```python
from build123d import *

# Parameters (mm, degrees)
F0_R     = 3.6
F0_R_2   = 11.05
F1_DEPTH = 6.5


# Not quite as in the source:
# - a feature names something its author has since deleted; it is built from what else it names


with BuildPart() as f1:
    # F0 (on Top) → F1 (new body)
    with BuildSketch(Plane.XY):
        with BuildLine():
            ThreePointArc((-23.0209464524, -29.3076083822), (-19.9383676627, -26.8167802289), (-17.6773098575, -23.5619170235))
            ThreePointArc((-17.6773098575, -23.5619170235), (-20.4709038775, -26.3215082368), (-23.0209464524, -29.3076083822))
        make_face()
        with BuildLine():
            ThreePointArc((-2.5600533635, -14.3957456382), (-1.63787321, -14.0667717582), (-0.7089513801, -13.7573460272))
            ThreePointArc((-0.7089513801, -13.7573460272), (-3.7381834506, -13.2395644299), (-6.5814605839, -12.0733226612))
            Line((-6.5814605839, -12.0733226612), (-2.5600533635, -14.3957456382))
        make_face()
        with BuildLine():
            ThreePointArc((-0.7089513801, -13.7573460272), (3.2568779095, -13.4262355322), (6.9693155956, -11.9926238203))
            ThreePointArc((6.9693155956, -11.9926238203), (3.0926272048, -12.7115843783), (-0.7089513801, -13.7573460272))
        make_face()
        with BuildLine():
            ThreePointArc((29.002813969, -3.3554863963), (22.1605329653, -5.9872334975), (17.5863384821, -11.7160769207))
            ThreePointArc((17.5863384821, -11.7160769207), (17.1389450218, -21.6742013703), (23.4307313902, -29.4058136055))
            ThreePointArc((23.4307313902, -29.4058136055), (37.4314802249, -29.4071108103), (44.4322291397, -17.282322802))
            ThreePointArc((44.4322291397, -17.282322802), (39.8127458528, -6.8897337985), (29.002813969, -3.3554863963))
        make_face()
        with Locations((24.2079713773, -13.6886037443)):
            Circle(F0_R, mode=Mode.SUBTRACT)
        with Locations((36.4874702709, -20.9787380615)):
            Circle(F0_R, mode=Mode.SUBTRACT)
        with Locations((33.9983616409, -11.0225966846)):
            Circle(F0_R, mode=Mode.SUBTRACT)
        with BuildLine():
            ThreePointArc((-23.0209464524, -29.3076083822), (-20.4709038775, -26.3215082368), (-17.6773098575, -23.5619170235))
            ThreePointArc((-17.6773098575, -23.5619170235), (-16.5669328393, -20.5090534106), (-16.1900430763, -17.2824658218))
            ThreePointArc((-16.1900430763, -17.2824658218), (-16.8601676515, -13.0029306649), (-18.8063889562, -9.1330843193))
            ThreePointArc((-18.8063889562, -9.1330843193), (-27.0153338433, -3.6471725985), (-36.8032431016, -4.9428716054))
            ThreePointArc((-36.8032431016, -4.9428716054), (-42.3755818337, -24.1754075155), (-23.0209464524, -29.3076083822))
        make_face()
        with Locations((-26.552398323, -23.5003339555)):
            Circle(F0_R, mode=Mode.SUBTRACT)
        with Locations((-36.419223994, -20.6778945734)):
            Circle(F0_R, mode=Mode.SUBTRACT)
        with Locations((-23.9660330315, -13.6886037443)):
            Circle(F0_R, mode=Mode.SUBTRACT)
        with BuildLine():
            ThreePointArc((-11.3063452022, 8.3060793433), (-9.4777201208, 10.4094594589), (-7.2686697166, 12.1089222888))
            Line((-7.2686697166, 12.1089222888), (-11.0034872924, 9.9526243561))
            ThreePointArc((-11.0034872924, 9.9526243561), (-11.1474831305, 9.1279846364), (-11.3063452022, 8.3060793433))
        make_face()
        with BuildLine():
            ThreePointArc((-13.8745275017, -0.137033899), (-12.3890775486, 4.023274448), (-11.3063452022, 8.3060793433))
            ThreePointArc((-11.3063452022, 8.3060793433), (-13.2731105164, 4.292175001), (-13.8745275017, -0.137033899))
        make_face()
        with BuildLine():
            ThreePointArc((6.7990177159, 12.5226532313), (9.6860598983, 9.0919172063), (12.891022892, 5.9561279205))
            ThreePointArc((12.891022892, 5.9561279205), (10.3843499056, 9.7397463301), (6.7990177159, 12.5226532313))
        make_face()
        with BuildLine():
            ThreePointArc((12.891022892, 5.9561279205), (13.810029624, 3.1522495359), (14.1209691729, 0.2180334624))
            Line((14.1209691729, 0.2180334624), (14.1209691729, 4.9018602452))
            ThreePointArc((14.1209691729, 4.9018602452), (13.5013908187, 5.4236214762), (12.891022892, 5.9561279205))
        make_face()
        with BuildLine():
            ThreePointArc((-11.4281301493, 27.3048605939), (-12.4782019744, 31.2955370079), (-13.8789707842, 35.1770310271))
            ThreePointArc((-13.8789707842, 35.1770310271), (-13.2461965273, 31.0564374771), (-11.4281301493, 27.3048605939))
        make_face()
        with BuildLine():
            ThreePointArc((6.7990177159, 12.5226532313), (10.3843499056, 9.7397463301), (12.891022892, 5.9561279205))
            ThreePointArc((12.891022892, 5.9561279205), (13.5013908187, 5.4236214762), (14.1209691729, 4.9018602452))
            Line((14.1209691729, 4.9018602452), (14.1209691729, 35.2180334624))
            ThreePointArc((14.1209691729, 35.2180334624), (4.2629861628, 21.8447879604), (-11.4281301493, 27.3048605939))
            ThreePointArc((-11.4281301493, 27.3048605939), (-10.3964763758, 18.6487931257), (-11.0034872924, 9.9526243561))
            Line((-11.0034872924, 9.9526243561), (-7.2686697166, 12.1089222888))
            ThreePointArc((-7.2686697166, 12.1089222888), (-0.2905931292, 14.2119827431), (6.7990177159, 12.5226532313))
        make_face()
        with BuildLine():
            ThreePointArc((6.9693155956, -11.9926238203), (12.2014668844, -6.8573870227), (14.1209691729, 0.2180334624))
            ThreePointArc((14.1209691729, 0.2180334624), (13.810029624, 3.1522495359), (12.891022892, 5.9561279205))
            ThreePointArc((12.891022892, 5.9561279205), (9.6860598983, 9.0919172063), (6.7990177159, 12.5226532313))
            ThreePointArc((6.7990177159, 12.5226532313), (-0.2905931292, 14.2119827431), (-7.2686697166, 12.1089222888))
            ThreePointArc((-7.2686697166, 12.1089222888), (-9.4777201208, 10.4094594589), (-11.3063452022, 8.3060793433))
            ThreePointArc((-11.3063452022, 8.3060793433), (-12.3890775486, 4.023274448), (-13.8745275017, -0.137033899))
            ThreePointArc((-13.8745275017, -0.137033899), (-11.8255695306, -7.0812961649), (-6.5814605839, -12.0733226612))
            ThreePointArc((-6.5814605839, -12.0733226612), (-3.7381834506, -13.2395644299), (-0.7089513801, -13.7573460272))
            ThreePointArc((-0.7089513801, -13.7573460272), (3.0926272048, -12.7115843783), (6.9693155956, -11.9926238203))
        make_face()
        with Locations((0.1209691729, 0.2180334624)):
            Circle(F0_R_2, mode=Mode.SUBTRACT)
        with BuildLine():
            ThreePointArc((-13.8745275017, -0.137033899), (-13.2731105164, 4.292175001), (-11.3063452022, 8.3060793433))
            ThreePointArc((-11.3063452022, 8.3060793433), (-11.1474831305, 9.1279846364), (-11.0034872924, 9.9526243561))
            Line((-11.0034872924, 9.9526243561), (-36.8032431016, -4.9428716054))
            ThreePointArc((-36.8032431016, -4.9428716054), (-27.0153338433, -3.6471725985), (-18.8063889562, -9.1330843193))
            ThreePointArc((-18.8063889562, -9.1330843193), (-16.0908458514, -4.7719029024), (-13.8745275017, -0.137033899))
        make_face()
        with BuildLine():
            Line((-2.5600533635, -14.3957456382), (-6.5814605839, -12.0733226612))
            ThreePointArc((-6.5814605839, -12.0733226612), (-11.8255695306, -7.0812961649), (-13.8745275017, -0.137033899))
            ThreePointArc((-13.8745275017, -0.137033899), (-16.0908458514, -4.7719029024), (-18.8063889562, -9.1330843193))
            ThreePointArc((-18.8063889562, -9.1330843193), (-16.8601676515, -13.0029306649), (-16.1900430763, -17.2824658218))
            ThreePointArc((-16.1900430763, -17.2824658218), (-16.5669328393, -20.5090534106), (-17.6773098575, -23.5619170235))
            ThreePointArc((-17.6773098575, -23.5619170235), (-10.5596558993, -18.2515569705), (-2.5600533635, -14.3957456382))
        make_face()
        with BuildLine():
            ThreePointArc((17.5863384821, -11.7160769207), (12.2698816763, -11.5493167715), (6.9693155956, -11.9926238203))
            ThreePointArc((6.9693155956, -11.9926238203), (3.2568779095, -13.4262355322), (-0.7089513801, -13.7573460272))
            ThreePointArc((-0.7089513801, -13.7573460272), (-1.63787321, -14.0667717582), (-2.5600533635, -14.3957456382))
            Line((-2.5600533635, -14.3957456382), (23.4307313902, -29.4058136055))
            ThreePointArc((23.4307313902, -29.4058136055), (17.1389450218, -21.6742013703), (17.5863384821, -11.7160769207))
        make_face()
        with BuildLine():
            Line((14.1209691729, 4.9018602452), (14.1209691729, 0.2180334624))
            ThreePointArc((14.1209691729, 0.2180334624), (12.2014668844, -6.8573870227), (6.9693155956, -11.9926238203))
            ThreePointArc((6.9693155956, -11.9926238203), (12.2698816763, -11.5493167715), (17.5863384821, -11.7160769207))
            ThreePointArc((17.5863384821, -11.7160769207), (22.1605329653, -5.9872334975), (29.002813969, -3.3554863963))
            ThreePointArc((29.002813969, -3.3554863963), (21.1797290943, 0.0844326658), (14.1209691729, 4.9018602452))
        make_face()
        with BuildLine():
            ThreePointArc((-11.4281301493, 27.3048605939), (4.2629861628, 21.8447879604), (14.1209691729, 35.2180334624))
            ThreePointArc((14.1209691729, 35.2180334624), (0.1004679333, 49.2180184516), (-13.8789707842, 35.1770310271))
            ThreePointArc((-13.8789707842, 35.1770310271), (-12.4782019744, 31.2955370079), (-11.4281301493, 27.3048605939))
        make_face()
        with Locations((0.1209691729, 28.0313078757)):
            Circle(F0_R, mode=Mode.SUBTRACT)
        with Locations((-7.0830557993, 35.1770310271)):
            Circle(F0_R, mode=Mode.SUBTRACT)
        with Locations((0.2946612417, 42.3107330219)):
            Circle(F0_R, mode=Mode.SUBTRACT)
    extrude(amount=F1_DEPTH)


solid = f1.part
```
CAD build for the part. Positions are in the model's coordinates, mm. A direction names the side the tool comes from. Coordinates: 2 decimals unless noted, no trailing zeros. Order: outer loops, then holes, each group sorted by start corner. A loop starts at its lowest first (then second) coordinate and runs counter-clockwise, first axis right, second up. Notation, with made-up numbers: (-28, -21) - (27, -21) arc R33 ccw to (27, 15) - close; hole circle Ø11 at (-19.75, 73.25). An arc over 180 degrees is marked (long way). Answer in a Markdown table with one row per item.
1. Slice it at C-C, the plane x = -26.5. List the corners of the cut face in (y, z).
Answer:
| item | result |
|---|---|
| outline | (-30.79, 0) - (-27.1, 0) - (-27.1, 6.5) - (-30.79, 6.5) - close; (-19.9, 0) - (-16.25, 0) - (-16.25, 6.5) - (-19.9, 6.5) - close; (-11.13, 0) - (1.01, 0) - (1.01, 6.5) - (-11.13, 6.5) - close |
2. Flat gauge pins, fed straight in: P1, Ø11.5, axis at x = -36.42, y = -20.68, coming from the -Z side; P2, Ø1.5, axis at x = 23, z = 2.5, coming from the +Y side; P3, Ø2, axis at y = 35.5, z = 4.5, coming from the +X side. Where does each tip first touch, or does it go through?
Answer:
| item | result |
|---|---|
| P1 | z = 0 |
| P2 | y = -0.49 |
| P3 | x = 14.12 |
3. Slice it at A-A, the plane x = 10. List the corners of the cut face in (y, z).
Answer:
| item | result |
|---|---|
| outline | (-21.65, 0) - (-4.73, 0) - (-4.73, 6.5) - (-21.65, 6.5) - close; (5.17, 0) - (45.14, 0) - (45.14, 6.5) - (5.17, 6.5) - close |
4. Slice it at B-B, the plane y = 41. List the corners of the cut face in (x, z), then the cut area to 3 significant figures.
Answer:
| item | result |
|---|---|
| outline | (-12.63, 0) - (-3.06, 0) - (-3.06, 6.5) - (-12.63, 6.5) - close; (3.65, 0) - (12.87, 0) - (12.87, 6.5) - (3.65, 6.5) - close |
| area | 122 mm² |
5. Pull direction Y, two halves, no side cores. Call faces 4 (the face through (21.28, 0.03, 3.2)), 5 (the face through (-39.276, -22.868, 3.204)), 6 (the face through (-10.67, -18.32, 3.2)), 7 (the face through (9, -8, 0)): +Y half, -Y half, draft (parallel to the pull), parting line (faces both ways), or undercut.
Answer:
| item | result |
|---|---|
| face 4 | +Y half |
| face 5 | undercut |
| face 6 | -Y half |
| face 7 | draft |
6. Drill centre lines: L1, parallel to Y at x = -8.5, z = 4.5; L2, parallel to X at y = -22, z = 6.25; L3, parallel to Y at x = -5.5, z = 4.5. Where is each one in solid material? Low to high. Write a range as from..to.
Answer:
| item | result |
|---|---|
| L1 | -17.07..-6.69, 7.13..31.87, 38.49..46.25 |
| L2 | -43.37..-39.77, -33.07..-29.82, -23.28..-15.86, 10.61..33.04, 39.94..43.61 |
| L3 | -15.6..-9.3, 9.73..31.94, 38.41..48.04 |
7. Slice it at D-D, the plane z = 5. Give the number of separate pieces and of enclosed holes in the cut face, then the cut area to 3 significant figures.
Answer:
| item | result |
|---|---|
| separate pieces | 1 |
| enclosed holes | 10 |
| area | 2,580 mm² |
8. 3-axis set-ups, long thin cutter, end or side, ignore diameter. For faces 1 (the face through (14.121, 20, 3)), 2 (the face through (2.23, 45.346, 3.204)), 3 (the face through (10.253, -21.796, 3.204)): which of +Z, -Z, +X, -X, +Y, -Y reach the whole face in a straight line?
Answer:
| item | result |
|---|---|
| face 1 | +Z, -Z, +X, +Y |
| face 2 | +Z, -Z |
| face 3 | +Z, -Z, -Y |
